For this review, take the finished solid that the model builds, in its own axes (mm). Round coordinates to 2 decimals unless told otherwise and drop trailing zeros. Write each loop counter-clockwise with the first axis right and the second up, starting at its lowest first coordinate (ties: lowest second). Pieces come first, ordered by that corner, then holes. Notation, with made-up numbers: (14, 79) -> (43, 79) arc R23 ccw to (43, 104) -> close; hole circle Ø8 at (81, -38). An arc over 180 degrees is marked (long way). Write each question's results on one line, items separated by ' | '. Start each with the question number.
Item 1: Add section C-C (x = 10). State the section outline as (y, z) points, plus the area to 4 significant figures.
Item 2: Add section A-A (y = 50). State the section outline as (x, z) points.
Item 3: Add section D-D (z = 1.55). State the section outline as (x, y) points, plus the area to 3 significant figures.
Item 4: Add section B-B (x = 30). State the section outline as (y, z) points.
Item 5: Clearance check with flat-ended pins moving along their axes: pin 1 (6 mm diameter, centred on x = 31.5, y = 21.5, fed in from -Z); pin 2 (1 mm diameter, centred on x = 50, y = 12, fed in from -Z). State where each tip first meets the part, or that it passes through.
Item 6: The part is to be moulded in two halves that separate along X. For faces 1 (the cylindrical face through (10.358, 52.727, 1.479)), 2 (the flat face through (39, 39, 1)), 3 (the cylindrical face through (32.747, 10.121, 1.479)), 4 (the flat face through (23, 23, 3)), say which applies: +X half, -X half, draft (parallel to the pull), parting line (faces both ways), or undercut.
Item 7: To check wall thickness, follow line 1 along Y through (x, z) = (10, 1.1); line 2 along X through (y, z) = (48, 1.7); line 3 along Y through (x, z) = (29, 0.25). State the ranges of each line that lie inside material, in increasing order.
from build123d import *

# Parameters (mm, degrees)
SCHIZZO1_W                   = 59
SCHIZZO1_H                   = 59
ESTRUSIONE_ESTRUSIONE1_DEPTH = 3
FORO_PER_VITE_M5_1_D         = 5.5
SMUSSO1_SIZE                 = 40


with BuildPart() as part:
    # Schizzo1 → Estrusione-Estrusione1 (new body)
    with BuildSketch(Plane.XY):
        with Locations((29.5, 29.5)):
            Rectangle(SCHIZZO1_W, SCHIZZO1_H)
    extrude(amount=ESTRUSIONE_ESTRUSIONE1_DEPTH)

    # Foro per Vite M5-1 (through all)
    with Locations(Plane.XY.offset(3)):
        with Locations((10, 10), (10, 30), (30, 10), (50, 10), (10, 50)):
            Hole(FORO_PER_VITE_M5_1_D / 2)

    # Smusso1
    smusso1_edges = [part.edges().sort_by_distance(p)[0] for p in [
        (59, 59, 1.5),
    ]]
    chamfer(smusso1_edges, length=SMUSSO1_SIZE)


solid = part.part
Responses:
1) outline: (0, 0) -> (7.25, 0) -> (7.25, 3) -> (0, 3) -> close; (12.75, 0) -> (27.25, 0) -> (27.25, 3) -> (12.75, 3) -> close; (32.75, 0) -> (47.25, 0) -> (47.25, 3) -> (32.75, 3) -> close; (52.75, 0) -> (59, 0) -> (59, 3) -> (52.75, 3) -> close | area: 127.5 mm^2
2) outline: (0, 0) -> (7.25, 0) -> (7.25, 3) -> (0, 3) -> close; (12.75, 0) -> (28, 0) -> (28, 3) -> (12.75, 3) -> close
3) outline: (0, 0) -> (59, 0) -> (59, 19) -> (19, 59) -> (0, 59) -> close; hole circle Ø5.5 at (10, 10); hole circle Ø5.5 at (10, 30); hole circle Ø5.5 at (10, 50); hole circle Ø5.5 at (30, 10); hole circle Ø5.5 at (50, 10) | area: 2,560 mm^2
4) outline: (0, 0) -> (7.25, 0) -> (7.25, 3) -> (0, 3) -> close; (12.75, 0) -> (48, 0) -> (48, 3) -> (12.75, 3) -> close
5) pin 1: stops at z = 0 | pin 2: passes through
6) face 1: undercut | face 2: +X half | face 3: undercut | face 4: draft
7) line 1: y = 0 to 7.25, 12.75 to 27.25, 32.75 to 47.25, 52.75 to 59 | line 2: x = 0 to 8.11, 11.89 to 30 | line 3: y = 0 to 7.44, 12.56 to 49
